Design review of the part built by this model. Coordinates are the model's own, in mm. Face numbers are marked on the shaded views. A direction names the side the tool comes from. Coordinates: 2 decimals unless noted, no trailing zeros. Order: outer loops, then holes, each group sorted by start corner. A loop starts at its lowest first (then second) coordinate and runs counter-clockwise, first axis right, second up. Notation, with made-up numbers: M 68,-9 L 117,-9 A16 cw 117,19 Z; hole C 32,22 d7. An arc over 180 degrees is marked long. Answer as a JSON object with one key per item and string values.
Autodesk Inventor part; units mm, degrees
ref_plane "Work Plane1" through (0, 0, -15) normal (0, 0, 1) x (1, 0, 0)
ref_plane "YZ Plane" through (0, 0, 0) normal (1, 0, 0) x (0, 1, 0)
ref_plane "XZ Plane" through (0, 0, 0) normal (0, 1, 0) x (-1, 0, 0)
sketch "Sketch1" plane through (0, 0, 0) normal (0, 0, 1) x (1, 0, 0)
  line L0 (0, 0) -> (25, 0)
  line L1 (25, 0) -> (25, 40)
  line L2 (25, 40) -> (0, 40)
  line L3 (0, 40) -> (0, 0)
  dimension "d1" = 25
  dimension "d2" = 40
  dimension "d3" = 25
extrude "Extrusion1" add sketch "Sketch1" against normal blind 30
sketch "Sketch2" plane through (25, 0, 0) normal (1, 0, 0) x (0, 0, -1)
  line L0 (0, 0) -> (30, 0)
  circle A0 centre (15, 6.56) radius 2.46
extrude "Extrusion2" cut sketch "Sketch2" against normal blind 30
sketch "Sketch3" plane through (0, 0, 0) normal (-1, 0, 0) x (0, 0, 1)
  line L0 (0, 0) -> (-30, 0)
  line L1 (-25.05, 0) -> (-4.95, 0)
  line L2 (-4.95, 0) -> (-4.95, 33.12)
  line L3 (-4.95, 33.12) -> (-25.05, 33.12)
  line L4 (-25.05, 33.12) -> (-25.05, 0)
  dimension "d11" = 20.1
extrude "Extrusion3" cut sketch "Sketch3" against normal blind 20
sketch "Sketch4" plane through (0, 0, 0) normal (0, -1, 0) x (1, 0, 0)
  line L0 (20, -4.95) -> (20, -25.05)
  line L1 (20, -15) -> (25, -15)
  line L2 (25, 0) -> (25, -30)
  line L3 (20, -8.025) -> (25, -8.025)
  line L4 (25, -8.025) -> (25, -21.975)
  line L5 (25, -21.975) -> (20, -21.975)
  line L6 (20, -21.975) -> (20, -8.025)
  line L7 (20, -8.025) -> (25, -21.975) construction
  line L8 (25, -8.025) -> (20, -21.975) construction
  line L9 (25, -12.54) -> (25, -17.46)
  point P0 (0, 0)
  point P1 (22.5, -15)
  dimension "d14" = 13.95
extrude "Extrusion4" add sketch "Sketch4" along normal blind 15
sketch "Sketch5" plane through (20, 0, 0) normal (-1, 0, 0) x (0, 0, 1)
  circle A0 centre (-15, 6.56) radius 2.46
  circle A1 centre (-15, 6.56) radius 4.7025
  circle A2 centre (-15, 6.56) radius 2.46
  circle A3 centre (-15, 6.56) radius 2.46
  point P0 (0, 0)
  dimension "d17" = 9.405
extrude "Extrusion5" cut sketch "Sketch5" against normal blind 2.1
sketch "Sketch6" plane through (25, 0, 0) normal (1, 0, 0) x (0, 0, -1)
  circle A0 centre (15, 6.56) radius 4.7025
  line L0 (15, 6.56) -> (15, 23.56)
  circle A1 centre (15, 23.56) radius 2.46
  point P0 (0, 0)
  dimension "d20" = 17
  dimension "d21" = 4.92
extrude "Extrusion6" cut sketch "Sketch6" against normal blind 10 contours A1
sketch "Sketch7" plane through (20, 0, 0) normal (-1, 0, 0) x (0, 0, 1)
  circle A0 centre (-15, 23.56) radius 2.46
  circle A1 centre (-15, 23.56) radius 4.7025
  point P0 (0, 0)
  dimension "d24" = 9.405
extrude "Extrusion7" cut sketch "Sketch7" against normal blind 2.1
sketch "Sketch9" plane through (25, 0, 0) normal (1, 0, 0) x (0, 0, -1)
  circle A0 centre (15, 6.56) radius 2.46
  circle A1 centre (15, 6.56) radius 2.46
  circle A2 centre (15, 23.56) radius 2.46
  circle A3 centre (15, 23.56) radius 2.46
  line L0 (30, 40) -> (30, 0)
  line L1 (30, 0) -> (30, 40)
  line L2 (30, 40) -> (0, 40)
  line L3 (0, 40) -> (0, 0)
  line L4 (0, 0) -> (8.025, 0)
  line L5 (21.975, 0) -> (21.975, -15)
  line L6 (21.975, -15) -> (8.025, -15)
  line L7 (8.025, -15) -> (8.025, 0)
  line L8 (0, 0) -> (8.025, 0)
  line L9 (21.975, 0) -> (30, 0)
extrude "Extrusion8" add sketch "Sketch9" along normal blind 5
sketch "Sketch10" plane through (0, 40, 0) normal (0, 1, 0) x (1, 0, 0)
  line L0 (0, 30) -> (30, 30)
  line L1 (30, 0) -> (0, 0)
  line L2 (0, 30) -> (30, 30)
  line L3 (30, 30) -> (30, 0)
  line L4 (30, 0) -> (0, 0)
  line L5 (0, 0) -> (0, 30)
extrude "Extrusion9" add sketch "Sketch10" along normal blind 30
sketch "Sketch12" plane through (30, 0, 0) normal (1, 0, 0) x (0, 0, -1)
  circle A0 centre (15, 6.56) radius 2.46
  line L0 (15, 6.56) -> (15, 15.06)
  circle A1 centre (15, 15.06) radius 2.525
  point P0 (0, 0)
  dimension "d31" = 8.5
  dimension "d33" = 5.05
extrude "Extrusion10" cut sketch "Sketch12" against normal blind 30 contours A1
sketch "Sketch15" plane through (0, 0, -25.05) normal (-1, 0, 0) x (0, 0, 1)
  line L0 (0, 33.12) -> (20.1, 33.12)
  line L1 (20.1, 33.12) -> (20.1, 0)
  line L2 (0, 33.12) -> (20.1, 33.12)
  line L3 (20.1, 33.12) -> (20.1, 31.1)
  line L4 (20.1, 31.1) -> (0, 31.1)
  line L5 (0, 31.1) -> (0, 33.12)
  point P0 (25.05, 0)
  dimension "d57" = 2.02
extrude "Extrusion13" add sketch "Sketch15" against normal blind 20
sketch "Sketch17" plane through (0, 0, 0) normal (0, 0, 1) x (1, 0, 0)
  line L0 (0, 70) -> (30, 70)
  line L1 (30, 70) -> (50.0622, 90.0622)
  line L2 (30, 70) -> (80, 70) construction
  line L3 (11.9522, 97.2454) -> (0, 85.2932)
  line L4 (0, 70) -> (0, 85.2932)
  line L5 (0, 70) -> (0, 0)
  line L6 (0, 70) -> (30, 70)
  line L7 (10.923, 112.2849) -> (0, 120.567)
  line L8 (50.0622, 105.3553) -> (50.0622, 120.567)
  line L9 (50.0622, 105.3553) -> (50.0622, 90.0622)
  arc A0 (11.9522, 97.2454) -> (10.923, 112.2849) centre (4.8811, 104.3165) ccw
  line L10 (4, 138.567) -> (0, 140.567)
  line L11 (4, 122.567) -> (0, 120.567)
  line L12 (4, 122.567) -> (8, 130.567)
  line L13 (4, 138.567) -> (8, 130.567)
  line L14 (0, 140.567) -> (30, 140.567)
  line L15 (30, 140.567) -> (50.0622, 120.567)
  dimension "d61" = 45
  dimension "d62" = 32.0271
  dimension "d72" = 10
extrude "Extrusion14" add sketch "Sketch17" against normal blind 30
sketch "Sketch21" plane through (0, 0, 0) normal (0, 0, 1) x (1, 0, 0)
  line L0 (50.0622, 90.0622) -> (30, 70)
  line L1 (30, 70) -> (50.0622, 90.0622)
  line L2 (50.0622, 90.0622) -> (50.0622, 120.567)
  line L3 (50.0622, 90.0622) -> (50.0622, 120.567)
  line L4 (0, 140.567) -> (30, 140.567)
  line L5 (50.0622, 120.567) -> (30, 140.567)
  line L6 (30, 140.567) -> (0, 140.567)
  line L7 (4, 138.567) -> (0, 140.567)
  line L8 (0, 140.567) -> (4, 138.567)
  line L9 (8, 130.567) -> (4, 138.567)
  line L10 (4, 138.567) -> (8, 130.567)
  line L11 (4, 122.567) -> (8, 130.567)
  line L12 (8, 130.567) -> (4, 122.567)
  line L13 (0, 120.567) -> (4, 122.567)
  line L14 (4, 122.567) -> (0, 120.567)
  line L15 (10.923, 112.2849) -> (0, 120.567)
  line L16 (0, 120.567) -> (10.923, 112.2849)
  line L17 (0, 85.2932) -> (11.9522, 97.2454)
  line L18 (11.9522, 97.2454) -> (0, 85.2932)
  line L19 (0, 85.2932) -> (0, 55.2932)
  line L20 (0, 55.2932) -> (30, 55.2932)
  line L21 (30, 55.2932) -> (30, 70)
  arc A0 (11.9522, 97.2454) -> (10.923, 112.2849) centre (4.8811, 104.3165) ccw
  dimension "d79" = 30
  dimension "d81" = 30
extrude "Extrusion15" add sketch "Sketch21" along normal blind 15
ref_plane "Work Plane1" through (0, 0, -15) normal (0, 0, 1) x (1, 0, 0)
mirror "Mirror1" about plane through (0, 0, -15) normal (0, 0, 1) of "Extrusion15"
properties part number "rec_c_16mm_x_60mm"
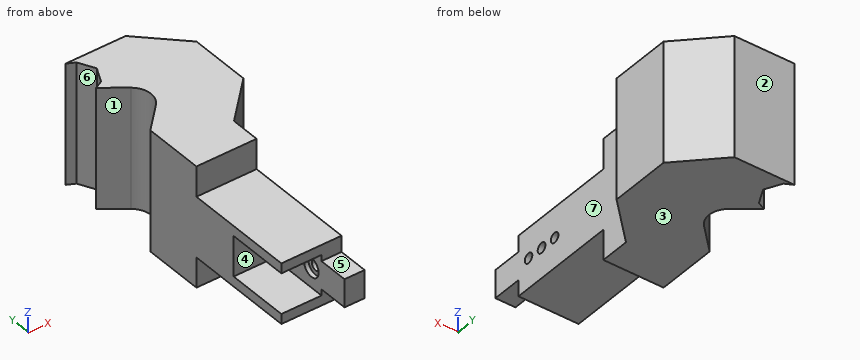
1) Add section A-A (y = 6.56). State the section outline as (x, z) points, and give its area (3 significant figures).
Taken from the geometry:
{"outline": "M 0,-30 L 30,-30 L 30,-17.46 L 22.1,-17.46 L 22.1,-19.7 L 20,-19.7 L 20,-25.05 L 0,-25.05 Z; M 0,-4.95 L 20,-4.95 L 20,-10.3 L 22.1,-10.3 L 22.1,-12.54 L 30,-12.54 L 30,0 L 0,0 Z", "area": "439 mm2"}
2) Add section C-C (x = 17). State the section outline as (y, z) points, and give its area (3 significant figures).
Taken from the geometry:
{"outline": "M 0,-30 L 55.29,-30 L 55.29,-45 L 140.57,-45 L 140.57,15 L 55.29,15 L 55.29,0 L 0,0 L 0,-4.95 L 31.1,-4.95 L 31.1,-25.05 L 0,-25.05 Z", "area": "6,150 mm2"}
3) Insertion check: pin 1 Ø1.5 at (y, z) = (112.5, -26) entering from -X; pin 2 Ø5 at (x, y) = (25, -6) entering from -Z (3 decimals); pin 3 Ø10 at (x, z) = (6, -29.5) entering from -Y. Each pin has a flat end and moves straight along its axis. Give the tip position at first contact, or say it passes through.
Taken from the geometry:
{"pin 1": "stops at x = 9.65", "pin 2": "stops at z = -21.975", "pin 3": "stops at y = 0"}
4) Add section B-B (z = -32). State the section outline as (x, y) points.
Taken from the geometry:
{"outline": "M 0,55.29 L 30,55.29 L 30,70 L 50.06,90.06 L 50.06,120.57 L 30,140.57 L 0,140.57 L 4,138.57 L 8,130.57 L 4,122.57 L 0,120.57 L 10.92,112.28 A10 cw 11.95,97.25 L 0,85.29 Z"}
5) To check wall thickness, follow L1, parallel to Y at x = 25.25, z = -15 (3 decimals); L2, parallel to Y at x = 21, z = -15 (1 decimal); L3, parallel to Y at x = 4, z = -12. State the ranges of each line that lie inside material, in increasing order.
Taken from the geometry:
{"L1": "y = -15 to 4.1, 9.02 to 12.535, 17.585 to 21.1, 26.02 to 140.567", "L2": "y = -15 to 1.9, 11.3 to 12.5, 17.6 to 18.9, 28.3 to 140.6", "L3": "y = 31.1 to 89.29, 117.53 to 122.57, 138.57 to 140.57"}
6) Mouldability with a two-part tool opening along Y and no side actions: class the marked faces 1, 2, 3 and 4 as released by +Y, released by -Y, zero draft, split by the parting line, or undercut.
Taken from the geometry:
{"face 1": "undercut", "face 2": "released by +Y", "face 3": "zero draft", "face 4": "released by -Y"}
7) Tool access review of the marked faces 5, 6 and 7: name each direction out of +Z, -Z, +X, -X, +Y, -Y from which nothing blocks a thin tool from reaching the whole face with its end or side.
Taken from the geometry:
{"face 5": "+Z, +X, -X, -Y", "face 6": "+Z, -Z, -X", "face 7": "+Z, -Z, +X, -Y"}
8) Add section D-D (z = -15). Count the separate pieces of the cut face and the enclosed holes in it, and give its area (3 significant figures).
Taken from the geometry:
{"separate pieces": "4", "enclosed holes": "0", "area": "4,160 mm2"}
